Verification items for the finished model (mm, model axes). A direction names the side the tool comes from. Coordinates: 2 decimals unless noted, no trailing zeros. Write each loop counter-clockwise with the first axis right and the second up, starting at its lowest first coordinate (ties: lowest second). Pieces come first, ordered by that corner, then holes. Notation, with made-up numbers: (-6.75, 52.5) - (32.25, 52.5) arc R24 cw to (32.25, 81.5) - close; hole circle Ø1 at (-40, 16). An arc over 180 degrees is marked (long way). Use one line per item in the form item = value. Start each with the question number.
(1) Sectioned sample at B-B (y = 2). Record the cut outline in (x, z).
(2) Mould release check, pull along Z, two halves, no side actions. Record for faces 1 (the cylindrical face through (29.472, -1.283, 0.07)), 2 (the cylindrical face through (-35.6, -2.97, -0.07)), 3 (the flat face through (-29, -7, -5)): released by +Z, released by -Z, zero draft, split by the parting line, or undercut.
(3) Material ranges on line 1 (Z direction, x = -34, y = -4.05); line 2 (X direction, y = 4.25, z = 0); line 3 (Y direction, x = -34, z = -3.75), recorded low to high. Write a range as [from, to].
(4) Sectioned sample at C-C (z = 0). Record the cut outline in (x, y), and give its area (3 significant figures).
(5) Tool access check on faces 4 (the flat face through (-32, 1, 0)), 5 (the flat face through (-36, -5, -1)), 6 (the flat face through (-38, -3, 0)), 7 (the flat face through (-36, 5, -1)). Record the directions out of +Z, -Z, +X, -X, +Y, -Y that give a thin tool (end or side, any length) a straight path to the whole face; none if there is none.
(6) Sectioned sample at A-A (x = 0). Record the cut outline in (y, z), and give its area (3 significant figures).
(7) Sectioned sample at D-D (z = -4). Record the cut outline in (x, y).
(8) Gauge pin test, flat ends, axial feed: pin 1 Ø1.5 at (x, z) = (-1, -1.5) entering from +Y; pin 2 Ø4.5 at (x, z) = (-34.5, 0) entering from -Y; pin 3 Ø3 at (x, z) = (-34, 0) entering from -Y; pin 4 Ø5 at (x, z) = (-36, 0.5) entering from +Y. Record the tip position at first contact, or that the pin passes through.
from build123d import *

# Parameters (mm, degrees)
SKETCH1_R               = 32
BOSS_EXTRUDE1_DEPTH     = 5
SKETCH4_W               = 38
SKETCH4_H               = 10
BOSS_EXTRUDE2_DEPTH     = 5
SKETCH5_R               = 29.5
SKETCH5_W               = 38
SKETCH5_H               = 2
CUT_EXTRUDE1_DEPTH      = 26.5
SKETCH6_R               = 1.6
CUT_EXTRUDE2_DEPTH      = 28
CUT_EXTRUDE2_DEPTH_BACK = 10


with BuildPart() as part:
    # Sketch1 → Boss-Extrude1 (new body, symmetric)
    with BuildSketch(Plane.XY):
        Circle(SKETCH1_R)
    extrude(amount=BOSS_EXTRUDE1_DEPTH, both=True)

    # Sketch4 → Boss-Extrude2 (add, symmetric)
    with BuildSketch(Plane.XY):
        with Locations((-19, 0)):
            Rectangle(SKETCH4_W, SKETCH4_H)
    extrude(amount=BOSS_EXTRUDE2_DEPTH, both=True)

    # Sketch5 → Cut-Extrude1 (cut)
    with BuildSketch(Plane.XY.offset(5)):
        Circle(SKETCH5_R)
        with Locations((-19, 0)):
            Rectangle(SKETCH5_W, SKETCH5_H)
    extrude(amount=-CUT_EXTRUDE1_DEPTH, mode=Mode.SUBTRACT)

    # Sketch6 → Cut-Extrude2 (cut, two sides)
    with BuildSketch(Plane(origin=(0, 5, 0), x_dir=(1, 0, 0), z_dir=(0, 1, 0))) as cut_extrude2_sk:
        with Locations((-34, 0)):
            Circle(SKETCH6_R)
    extrude(amount=CUT_EXTRUDE2_DEPTH, mode=Mode.SUBTRACT)
    extrude(cut_extrude2_sk.sketch, amount=-CUT_EXTRUDE2_DEPTH_BACK, mode=Mode.SUBTRACT)


solid = part.part
Answers below:
q1.outline = (-38, -5) - (-29.43, -5) - (-29.43, 5) - (-38, 5) - close; (29.43, -5) - (31.94, -5) - (31.94, 5) - (29.43, 5) - close; hole circle Ø3.2 at (-34, 0)
q2.face_1 = zero draft
q2.face_2 = undercut
q2.face_3 = released by -Z
q3.line_1 = [-5, -1.6], [1.6, 5]
q3.line_2 = [-38, -35.6], [-32.4, -29.19], [29.19, 31.72]
q3.line_3 = [-5, -1], [1, 5]
q4.outline = (-38, -5) - (-35.6, -5) - (-35.6, -1) - (-38, -1) - close; (-38, 1) - (-35.6, 1) - (-35.6, 5) - (-38, 5) - close; (-32.4, -5) - (-31.61, -5) arc R32 ccw (long way) to (-31.61, 5) - (-32.4, 5) - (-32.4, 1) - (-29.48, 1) arc R29.5 cw (long way) to (-29.48, -1) - (-32.4, -1) - close
q4.area = 502 mm2
q5.face_4 = +Z, -Z, -X
q5.face_5 = +Z, -Z, -X, -Y
q5.face_6 = +Z, -Z, -X, +Y, -Y
q5.face_7 = +Z, -Z, -X, +Y
q6.outline = (-32, -5) - (-29.5, -5) - (-29.5, 5) - (-32, 5) - close; (29.5, -5) - (32, -5) - (32, 5) - (29.5, 5) - close
q6.area = 50.0 mm2
q7.outline = (-38, -5) - (-31.61, -5) arc R32 ccw (long way) to (-31.61, 5) - (-38, 5) - (-38, 1) - (-29.48, 1) arc R29.5 cw (long way) to (-29.48, -1) - (-38, -1) - close
q8.pin_1 = 32
q8.pin_2 = -5
q8.pin_3 = through
q8.pin_4 = 5
